Autodesk Inventor part; units mm, degrees
ref_plane "Work Plane1" through (14.9, 0, 0) normal (1, 0, 0) x (0, 1, 0)
ref_plane "XZ Plane" through (0, 0, 0) normal (0, 1, 0) x (-1, 0, 0)
ref_plane "XY Plane" through (0, 0, 0) normal (0, 0, 1) x (1, 0, 0)
sketch "Sketch1" plane through (0, 0, 0) normal (0, 0, 1) x (1, 0, 0)
  circle A0 centre (0, 0) radius 14.89
  circle A1 centre (0, 0) radius 6
  circle A2 centre (0, 0) radius 3.175
  dimension "d0" = 29.78
  dimension "d1" = 12
  dimension "d41" = 6.35
extrude "Extrusion1" add sketch "Sketch1" along normal blind 25 contours A0 | A1
sketch "Sketch2" plane through (0, 0, 25) normal (0, 0, 1) x (1, 0, 0)
  circle A0 centre (0, 0) radius 14.89
  circle A1 centre (0, 0) radius 9
  circle A2 centre (0, 0) radius 14.89
  line L0 (-3.6007, 8.2483) -> (-5.9571, 13.6464)
  line L1 (5.9571, 13.6464) -> (3.6007, 8.2483)
  line L2 (-5.3429, -7.2425) -> (-8.8396, -11.9822)
  line L3 (-14.7967, -1.6642) -> (-8.9436, -1.0059)
  line L4 (8.9436, -1.0059) -> (14.7967, -1.6642)
  line L5 (8.8396, -11.9822) -> (5.3429, -7.2425)
  dimension "d14" = 18
  dimension "d24" = 360
extrude "Extrusion2" cut sketch "Sketch2" against normal blind 10.5 contours A0 L4 A1 L1 | L0 A1 L3 A0 | A1 | A0 L2 A1 L5
ref_plane "Work Plane1" through (14.9, 0, 0) normal (1, 0, 0) x (0, 1, 0)
sketch "Sketch3" plane through (14.9, 0, 0) normal (1, 0, 0) x (0, 1, 0)
  line L0 (-1.6642, 14.5) -> (-1.6642, 25)
  line L1 (-11.9822, 25) -> (-1.6642, 25)
  line L2 (-11.9822, 25) -> (-11.9822, 14.5)
  line L3 (-11.9822, 14.5) -> (-11.9822, 14.5)
  line L4 (-11.9822, 14.5) -> (-11.9822, 25)
  line L5 (-1.6642, 25) -> (-11.9822, 25)
  line L6 (-1.6642, 25) -> (-1.6642, 14.5)
  line L7 (-1.6642, 14.5) -> (13.6464, 14.5)
  line L8 (13.6464, 14.5) -> (13.6464, 25)
  line L9 (13.6464, 25) -> (13.6464, 25)
  line L10 (13.6464, 25) -> (13.6464, 14.5)
  line L11 (13.6464, 14.5) -> (-1.6642, 14.5)
  line L12 (14.89, 0) -> (-14.89, 0)
  line L13 (14.89, 25) -> (13.6464, 25)
  line L14 (14.89, 25) -> (14.89, 0)
  line L15 (14.89, 0) -> (14.89, 25)
  line L16 (-14.89, 0) -> (-14.89, 14.5)
  line L17 (14.89, 0) -> (-14.89, 0)
  line L18 (-14.89, 14.5) -> (-14.89, 0)
  line L19 (-7.89, 0) -> (-14.89, 0)
  line L20 (-14.89, 0) -> (-14.89, 14.5)
  line L21 (-14.89, 7.25) -> (-7.89, 7.25)
  circle A0 centre (-11.39, 7.25) radius 3.5
  circle A1 centre (-11.39, 7.25) radius 1.75
  point P0 (0, 0)
  dimension "d27" = 29.78
  dimension "d30" = 3.5
extrude "Extrusion3" cut sketch "Sketch3" against normal blind 10
extrude "Extrusion4" cut sketch "Sketch3" against normal blind 30 contours A1 L21 | L21 A1
sketch "Sketch4" plane through (0, 0, 0) normal (0, 0, -1) x (-1, 0, 0)
  arc A0 (-8.8396, -11.9822) -> (8.8396, -11.9822) centre (0, 0) ccw
  line L0 (0, 0) -> (-0.5, 0)
  line L1 (-0.5, 0) -> (-0.5, -14.8816)
  line L2 (0, 0) -> (0.5, 0)
  line L3 (0.5, 0) -> (0.5, -14.8816)
  line L4 (-0.5, 0) -> (-0.5, 14.8816)
  line L5 (0.5, 0) -> (0.5, 14.8816)
  arc A1 (5.3429, -7.2425) -> (8.9436, -1.0059) centre (0, 0) ccw
  circle A2 centre (0, 0) radius 14.89
  point P0 (-8.8396, 11.9822)
  dimension "d33" = 0.5
  dimension "d34" = 0.5
extrude "Extrusion5" cut sketch "Sketch4" against normal blind 15 contours L1 L0 L2 L3 A0
sketch "Sketch5" plane through (-0.5, -14.8816, 0) normal (1, 0, 0) x (0, 0, -1)
  line L0 (0, 0) -> (-14.5, 0)
  line L1 (-14.5, 0) -> (-14.5, 2.8994)
  line L2 (-14.5, 2.8994) -> (-25, 2.8994)
  line L3 (-25, 13.2174) -> (-25, 2.8994)
  line L4 (-25, 13.2174) -> (-14.5, 13.2174)
  line L5 (-14.5, 13.2174) -> (-14.5, 28.528)
  line L6 (-14.5, 28.528) -> (-25, 28.528)
  line L7 (-25, 28.528) -> (-25, 28.528)
  line L8 (-25, 28.528) -> (-14.5, 28.528)
  line L9 (-14.5, 28.528) -> (-14.5, 13.2174)
  line L10 (-14.5, 13.2174) -> (-25, 13.2174)
  line L11 (-25, 2.8994) -> (-25, 13.2174)
  line L12 (-25, 2.8994) -> (-14.5, 2.8994)
  line L13 (-14.5, 2.8994) -> (-14.5, 0)
  line L14 (-14.5, 0) -> (0, 0)
  line L15 (0, 0) -> (0, 0)
  line L16 (-4.9878, 0.8209) -> (-9.5122, 0.8209)
  line L17 (-14.5, 8.9025) -> (0, 8.9025)
  line L18 (0, 8.9025) -> (0, 8.9025)
  line L19 (0, 8.9025) -> (-14.5, 8.9025)
  line L20 (-14.5, 8.9025) -> (-14.5, 8.9025)
  line L21 (-14.5, 20.8816) -> (-14.5, 8.9025)
  line L22 (-14.5, 20.8816) -> (0, 20.8816)
  line L23 (0, 29.7716) -> (0, 0)
  line L24 (-14.5, 20.8816) -> (-14, 20.8816)
  line L25 (0, 29.7716) -> (0, 29.2716)
  line L26 (0, 29.2716) -> (-14, 20.8816)
  line L27 (-14.5, 20.8585) -> (0, 20.8585)
  line L28 (0, 8.9025) -> (0, 20.8816)
  line L29 (-14, 20.8816) -> (-14.0385, 20.8585)
  line L30 (-14.5, 18.0566) -> (0, 18.0566)
  line L31 (-14.5, 18.0566) -> (-14.5, 11.7462)
  line L32 (-14.5, 18.0145) -> (0, 18.0145)
  line L33 (-14.5, 18.0145) -> (-14, 18.0145)
  line L34 (-14, 18.0145) -> (0, 29.2716)
  point P0 (0, 14.8816)
  point P1 (-13.9476, 18.0566)
  dimension "d37" = 0.5
  dimension "d38" = 0.5
  dimension "d42" = 0.5
extrude "Extrusion6" cut sketch "Sketch5" along normal blind 1 contours L32 L34 L30 L23 | L30 L34 L27 L23 | L32 L5 L30 L34 | L27 L34 L22 L23 | L30 L5 L27 L34 | L22 L34 L23 | L27 L29 L22 L34 | L22 L26 L34
properties part number "PHAN NHOM 6"
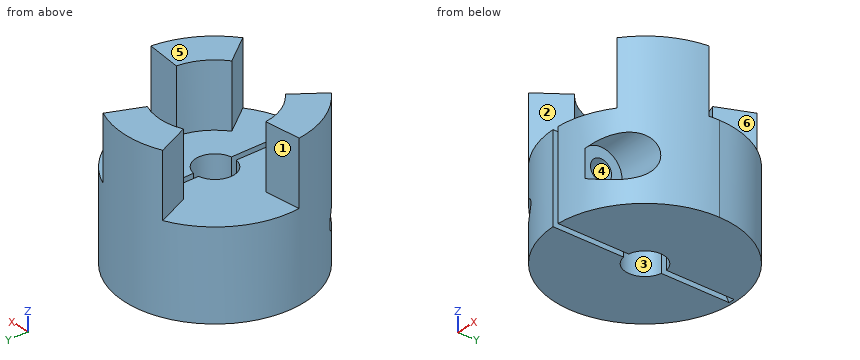
Geometry check sheet. Reference: the model listing, model coordinates, mm. Face numbers are marked on the shaded views. A direction names the side the tool comes from. Coordinates: 2 decimals unless noted, no trailing zeros. Order: outer loops, then holes, each group sorted by start corner. A loop starts at its lowest first (then second) coordinate and runs counter-clockwise, first axis right, second up. Notation, with made-up numbers: (77.5, 87.5) - (129.5, 87.5) arc R18 ccw to (129.5, 95.5) - close; hole circle Ø1 at (21.5, -22.75). An arc over 180 degrees is marked (long way). Answer as a JSON object with one key per item and string values. Group by question number.
Item 1: Depth check by flat-ended pin: pin 1 Ø4 at (y, z) = (-11.39, 7.25) entering from +X; pin 2 Ø5.5 at (y, z) = (-11.39, 7.25) entering from -X; pin 3 Ø6 at (y, z) = (-6.5, 7.5) entering from -X. Enter the tip coordinate at first touch or a pass-through.
Item 2: Tool access check on the marked faces 1, 2 and 3. Record the directions out of +Z, -Z, +X, -X, +Y, -Y that give a thin tool (end or side, any length) a straight path to the whole face; none if there is none.
Item 3: Sectioned sample at A-A, the plane y = 2. Record the cut outline in (x, z), and give its area (3 significant figures).
Item 4: Draft check along Z on the marked faces 4, 5 and 6. Enter one of: +Z half, -Z half, draft (parallel to the pull), parting line (faces both ways), or undercut.
Item 5: Sectioned sample at B-B, the plane z = 23. Record the cut outline in (x, y), and give its area (3 significant figures).
Item 6: Scan lines: probe 1 along Z at (x, y) = (3.15, -11.39); probe 2 along Z at (x, y) = (8.5, -11.39); probe 3 along Z at (x, y) = (-6.5, 8.5). Record each from-to range of solid material in increasing order.
Item 7: Sectioned sample at D-D, the plane y = -11.25. Record the cut outline in (x, z), and give its area (3 significant figures).
Item 8: Sectioned sample at C-C, the plane x = 0. Record the cut outline in (y, z), and give its area (3 significant figures).
Resolved:
{
 "1": {"pin 1": "x = 4.9", "pin 2": "x = -12.13", "pin 3": "x = -14.47"},
 "2": {"face 1": "+Z, -X, +Y", "face 2": "+Z, -Y", "face 3": "+Z, -Z"},
 "3": {"outline": "(-14.76, 0) - (-2.47, 0) - (-2.47, 14.5) - (-14.76, 14.5) - close; (2.47, 0) - (14.76, 0) - (14.76, 14.5) - (2.47, 14.5) - close", "area": "356 mm^2"},
 "4": {"face 4": "undercut", "face 5": "+Z half", "face 6": "draft"},
 "5": {"outline": "(-14.8, -1.66) arc R14.89 ccw to (-8.84, -11.98) - (-5.34, -7.24) arc R9 cw to (-8.94, -1.01) - close; (-5.96, 13.65) - (-3.6, 8.25) arc R9 cw to (3.6, 8.25) - (5.96, 13.65) arc R14.89 ccw to start; (5.34, -7.24) - (8.84, -11.98) arc R14.89 ccw to (14.8, -1.66) - (8.94, -1.01) arc R9 cw to start", "area": "174 mm^2"},
 "6": {"probe 1": "0 to 5.5, 9 to 14.5", "probe 2": "0 to 3.75, 10.75 to 25", "probe 3": "0 to 14.5"},
 "7": {"outline": "(-9.75, 0) - (-0.5, 0) - (-0.5, 5.51) - (-9.75, 5.51) - close; (-9.75, 8.99) - (-0.5, 8.99) - (-0.5, 14.5) - (-8.3, 14.5) - (-8.3, 25) - (-9.75, 25) - close; (0.5, 0) - (9.75, 0) - (9.75, 3.75) - (4.9, 3.75) - (4.9, 5.51) - (0.5, 5.51) - close; (0.5, 8.99) - (4.9, 8.99) - (4.9, 10.75) - (9.75, 10.75) - (9.75, 25) - (8.3, 25) - (8.3, 14.5) - (0.5, 14.5) - close", "area": "217 mm^2"},
 "8": {"outline": "(5.98, 14.04) - (6, 14) - (14.39, 0) - (14.89, 0) - (14.89, 25) - (9, 25) - (9, 14.5) - (5.98, 14.5) - close", "area": "132 mm^2"}
}
